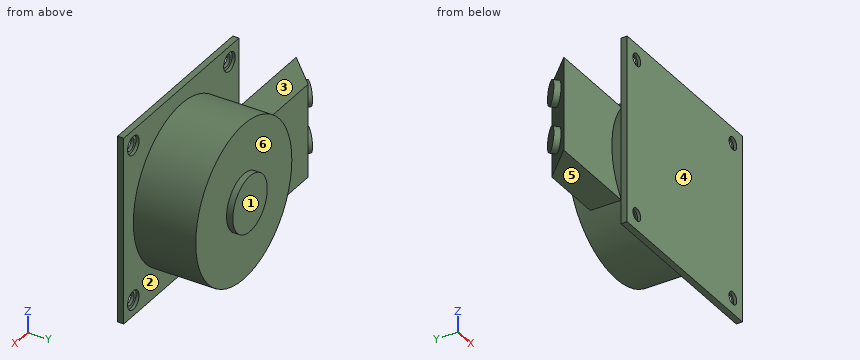
from build123d import *

# Parameters (mm, degrees)
SKETCH_1_W               = 300
SKETCH_1_H               = 300
EXTRUDE_1_DEPTH          = 10
SKETCH_2_R               = 125
EXTRUDE_2_DEPTH          = 100
SKETCH_3_W               = 150
SKETCH_3_H               = 50
EXTRUDE_3_DEPTH          = 200
DRAFT_3_ANGLE            = 45
SKETCH_5_R               = 18.8
EXTRUDE_5_DEPTH          = 10
SKETCH_6_R               = 44.85
EXTRUDE_6_DEPTH          = 10
SKETCH_7_R               = 15
CUT_EXTRUDE_1_DEPTH      = 5
SKETCH_8_R               = 10
CUT_EXTRUDE_2_DEPTH      = 25
MIRROR_2_COPY_1_SKETCH_R = 15
MIRROR_2_COPY_1_DEPTH    = 5
MIRROR_2_COPY_2_SKETCH_R = 10
MIRROR_2_COPY_2_DEPTH    = 25


with BuildPart() as part:
    # 草图1 → 凸台-拉伸1 (new body)
    with BuildSketch(Plane(origin=(0, 0, 0), x_dir=(1, 0, 0), z_dir=(0, 1, 0))):
        Rectangle(SKETCH_1_W, SKETCH_1_H)
    extrude(amount=EXTRUDE_1_DEPTH)

    # 草图2 → 凸台-拉伸2 (add)
    with BuildSketch(Plane(origin=(0, 10, 0), x_dir=(1, 0, 0), z_dir=(0, 1, 0))):
        Circle(SKETCH_2_R)
    extrude(amount=EXTRUDE_2_DEPTH)

    # 草图3 → 凸台-拉伸3 (add)
    with BuildSketch(Plane(origin=(0, 0, 0), x_dir=(0, 0, -1), z_dir=(1, 0, 0))):
        with Locations((0, 65)):
            Rectangle(SKETCH_3_W, SKETCH_3_H)
    extrude(amount=-EXTRUDE_3_DEPTH)

    # 拔模3
    draft_3_faces = [part.faces().sort_by_distance(p)[0] for p in [
        (-200, 65, 0),
    ]]
    draft(draft_3_faces, Plane(origin=(-200, 90, 75), x_dir=(0, 0, 1), z_dir=(0, 1, 0)), DRAFT_3_ANGLE)

    # 草图5 → 凸台-拉伸5 (add)
    with BuildSketch(Plane(origin=(-145, 145, 0), x_dir=(0, 0, 1), z_dir=(-0.707106781, 0.707106781, 0))):
        with Locations((-37.5, -113.13708499)):
            Circle(SKETCH_5_R)
        with Locations((37.5, -113.13708499)):
            Circle(SKETCH_5_R)
    extrude(amount=EXTRUDE_5_DEPTH)

    # 草图6 → 凸台-拉伸6 (add)
    with BuildSketch(Plane(origin=(0, 110, 0), x_dir=(1, 0, 0), z_dir=(0, 1, 0))):
        Circle(SKETCH_6_R)
    extrude(amount=EXTRUDE_6_DEPTH)

    # 草图7 → 切除-拉伸1 (cut)
    with BuildSketch(Plane(origin=(0, 10, 0), x_dir=(1, 0, 0), z_dir=(0, 1, 0))):
        with Locations((-125, 125)):
            Circle(SKETCH_7_R)
    cut_extrude_1 = extrude(amount=-CUT_EXTRUDE_1_DEPTH, mode=Mode.SUBTRACT)

    # 草图8 → 切除-拉伸2 (cut)
    with BuildSketch(Plane(origin=(0, 5, 0), x_dir=(1, 0, 0), z_dir=(0, 1, 0))):
        with Locations((-125, 125)):
            Circle(SKETCH_8_R)
    cut_extrude_2 = extrude(amount=-CUT_EXTRUDE_2_DEPTH, mode=Mode.SUBTRACT)

    # 镜向1: 切除-拉伸1, 切除-拉伸2 across plane
    add(cut_extrude_1.mirror(Plane.XY), mode=Mode.SUBTRACT)
    add(cut_extrude_2.mirror(Plane.XY), mode=Mode.SUBTRACT)

    # 镜向2: 切除-拉伸1, 切除-拉伸2 across plane
    add(cut_extrude_1.mirror(Plane(origin=(0, 0, 0), x_dir=(0, 0, 1), z_dir=(1, 0, 0))), mode=Mode.SUBTRACT)
    add(cut_extrude_2.mirror(Plane(origin=(0, 0, 0), x_dir=(0, 0, 1), z_dir=(1, 0, 0))), mode=Mode.SUBTRACT)

    # 镜向2 copy 1 sketch → 镜向2 copy 1 (cut)
    with BuildSketch(Plane(origin=(0, 10, 0), x_dir=(-1, 0, 0), z_dir=(0, 1, 0))):
        with Locations((-125, 125)):
            Circle(MIRROR_2_COPY_1_SKETCH_R)
    extrude(amount=-MIRROR_2_COPY_1_DEPTH, mode=Mode.SUBTRACT)

    # 镜向2 copy 2 sketch → 镜向2 copy 2 (cut)
    with BuildSketch(Plane(origin=(0, 5, 0), x_dir=(-1, 0, 0), z_dir=(0, 1, 0))):
        with Locations((-125, 125)):
            Circle(MIRROR_2_COPY_2_SKETCH_R)
    extrude(amount=-MIRROR_2_COPY_2_DEPTH, mode=Mode.SUBTRACT)


solid = part.part
Geometry: final body of the model. Coordinates: model frame, mm. Face numbers are marked on the shaded views. A direction names the side the tool comes from. Give positions to 0.01 mm unless a question says otherwise; leave off trailing zeros. Write each loop counter-clockwise with the first axis right and the second up, starting at its lowest first coordinate (ties: lowest second). Pieces come first, ordered by that corner, then holes.
(1) Cut plane C-C, the plane y = 15. Return loops of the section in (x, z).
(2) Ray query, line 1 (Z direction, x = 125, y = 1); line 2 (Y direction, x = -99.5, z = 134). Return the intervals inside material, ascending.
(3) Mould query, pull axis Y, two halves, no side actions, for the marked faces 1, 2 and 3. Classes: released by +Y, released by -Y, zero draft, split by the parting line, or undercut.
(4) Cut plane A-A, the plane x = 0. Return loops of the section in (y, z).
(5) First-contact query: P1, Ø25, axis at x = -208, y = 75.5, coming from the -Z side; P2, Ø2, axis at x = 37, z = -29, coming from the +Y side; P3, Ø8, axis at y = 7, z = 48, coming from the -X side. Flat tips, straight axial feed; report the tip coordinate or a pass-through.
(6) Cut plane B-B, the plane z = 0. Return loops of the section in (x, y), then the cut area to 3 significant figures.
(7) Cut plane D-D, the plane x = -155.5. Return loops of the section in (y, z).
(8) Access query for the marked faces 4, 5 and 6. Directions: +Z, -Z, +X, -X, +Y, -Y. A direction counts if a zero-diameter tool reaches every point of the face in a straight line with its end or side. Return the directions, or none.
Values follow:
1. outline: circle Ø250 at (0, 0)
2. line 1: z = -150 to -135, -115 to 115, 135 to 150
2. line 2: y = 0 to 10
3. face 1: released by +Y
3. face 2: undercut
3. face 3: zero draft
4. outline: (0, -150) - (10, -150) - (10, -125) - (110, -125) - (110, -44.85) - (120, -44.85) - (120, 44.85) - (110, 44.85) - (110, 125) - (10, 125) - (10, 150) - (0, 150) - close
5. P1: stops at z = -75
5. P2: stops at y = 110
5. P3: stops at x = -150
6. outline: (-250, 40) - (-125, 40) - (-125, 10) - (-150, 10) - (-150, 0) - (150, 0) - (150, 10) - (125, 10) - (125, 110) - (44.85, 110) - (44.85, 120) - (-44.85, 120) - (-44.85, 110) - (-125, 110) - (-125, 90) - (-200, 90) - close
6. area: 33,900 mm2
7. outline: (40, -75) - (90, -75) - (90, 75) - (40, 75) - close
8. face 4: +Z, -Z, +X, -X, -Y
8. face 5: -Z, -X, +Y
8. face 6: +Y
